Work out the finished part from the listing and answer in its coordinate system (mm). Round coordinates to 2 decimals unless told otherwise and drop trailing zeros. Write each loop counter-clockwise with the first axis right and the second up, starting at its lowest first coordinate (ties: lowest second). Pieces come first, ordered by that corner, then holes.
1. Straight lines are drawn through the part: probe 1 along Y at (x, z) = (0, -0.1); probe 2 along X at (y, z) = (7.5, -0.3); probe 3 along Y at (x, z) = (0.65, -0.05). For each, find the intervals that lie inside material, in ascending order.
2. Find section D-D (y = 5). Write down the section's boundary in (x, z), and give its area (3 significant figures).
3. A flat-ended cylindrical pin translates along its axis: pin 1 Ø0.5 at (y, z) = (6, 0) entering from +X. Find the tip coordinate at first contact, or state that the pin passes through.
4. Find section B-B (y = 0.5). Write down the section's boundary in (x, z), and give its area (3 significant figures).
5. Find section C-C (z = 0.4). Write down the section's boundary in (x, y), and give its area (3 significant figures).
6. Find section A-A (x = 0). Write down the section's boundary in (y, z).
```python
from build123d import *

# Parameters (mm, degrees)
SZKIC1_W                    = 1
SZKIC1_H                    = 1
DODANIE_WYCI_GNI_CIE2_DEPTH = 9.5
SZKIC2_R                    = 0.250044668
WYTNIJ_WYCI_GNI_CIE1_DEPTH  = 9.5
SZKIC3_W                    = 1
SZKIC3_H                    = 1.5
DODANIE_WYCI_GNI_CIE3_DEPTH = 0.5
SZKIC4_W                    = 1
SZKIC4_H                    = 1.498354428
DODANIE_WYCI_GNI_CIE4_DEPTH = 0.5
ZAOKR_GLENIE1_R             = 0.25
ZAOKR_GLENIE2_R             = 0.25


with BuildPart() as part:
    # Szkic1 → Dodanie-wyciągnięcie2 (new body)
    with BuildSketch(Plane(origin=(0, 0, 0), x_dir=(1, 0, 0), z_dir=(0, 1, 0))):
        Rectangle(SZKIC1_W, SZKIC1_H)
    extrude(amount=DODANIE_WYCI_GNI_CIE2_DEPTH)

    # Szkic2 → Wytnij-wyciągnięcie1 (cut)
    with BuildSketch(Plane(origin=(0, 0, -0.5), x_dir=(-1, 0, 0), z_dir=(0, 0, -1))):
        with Locations((0, 0.5)):
            Circle(SZKIC2_R)
    extrude(amount=-WYTNIJ_WYCI_GNI_CIE1_DEPTH, mode=Mode.SUBTRACT)

    # Szkic3 → Dodanie-wyciągnięcie3 (add)
    with BuildSketch(Plane(origin=(0.5, 0, 0), x_dir=(0, 0, -1), z_dir=(1, 0, 0))):
        with Locations((0, 8.75)):
            Rectangle(SZKIC3_W, SZKIC3_H)
    extrude(amount=DODANIE_WYCI_GNI_CIE3_DEPTH)

    # Szkic4 → Dodanie-wyciągnięcie4 (add)
    with BuildSketch(Plane.ZY.offset(0.5)):
        with Locations((0, 8.750822786)):
            Rectangle(SZKIC4_W, SZKIC4_H)
    extrude(amount=DODANIE_WYCI_GNI_CIE4_DEPTH)

    # Zaokrąglenie1
    zaokr_glenie1_edges = [part.edges().sort_by_distance(p)[0] for p in [
        (0, 9.5, -0.5),
        (0.75, 8, 0.5),
        (0.75, 8, -0.5),
        (1, 8.75, 0.5),
        (1, 8.75, -0.5),
        (1, 9.5, 0),
        (-0.75, 8.001645572, -0.5),
        (-1, 8.750822786, -0.5),
        (-1, 8.750822786, 0.5),
        (-1, 9.5, 0),
        (0, 9.5, 0.5),
    ]]
    fillet(zaokr_glenie1_edges, radius=ZAOKR_GLENIE1_R)

    # Zaokrąglenie2
    # the kernel refuses this fillet: 0.25 mm, written as the material it takes off along each edge
    with BuildSketch(Plane(origin=(0.75, 8.25, -0.25), x_dir=(0, -1, 0), z_dir=(1, 0, 0))) as zaokr_glenie2_piece_1_section:
        Polygon((0, 0), (ZAOKR_GLENIE2_R, 0), (ZAOKR_GLENIE2_R, ZAOKR_GLENIE2_R), (0, ZAOKR_GLENIE2_R), align=None)
    zaokr_glenie2_piece_1 = extrude(amount=ZAOKR_GLENIE2_R, mode=Mode.PRIVATE)
    zaokr_glenie2_piece_1 = zaokr_glenie2_piece_1 - Plane(origin=(0.75, 8.25, -0.25), x_dir=(0, 0.7071067811865475, 0.7071067811865475), z_dir=(1, 0, 0)) * Sphere(ZAOKR_GLENIE2_R, mode=Mode.PRIVATE)
    add(zaokr_glenie2_piece_1, mode=Mode.SUBTRACT)
    with BuildSketch(Plane(origin=(-0.75, 8.251645572, -0.25), x_dir=(0, -1, 0), z_dir=(-1, 0, 0))) as zaokr_glenie2_piece_2_section:
        Polygon((0, 0), (ZAOKR_GLENIE2_R, 0), (ZAOKR_GLENIE2_R, -ZAOKR_GLENIE2_R), (0, -ZAOKR_GLENIE2_R), align=None)
    zaokr_glenie2_piece_2 = extrude(amount=ZAOKR_GLENIE2_R, mode=Mode.PRIVATE)
    zaokr_glenie2_piece_2 = zaokr_glenie2_piece_2 - Plane(origin=(-0.75, 8.251645572, -0.25), x_dir=(0, 0.7071067811865475, 0.7071067811865475), z_dir=(-1, 0, 0)) * Sphere(ZAOKR_GLENIE2_R, mode=Mode.PRIVATE)
    add(zaokr_glenie2_piece_2, mode=Mode.SUBTRACT)
    with BuildSketch(Plane(origin=(0.75, 8.25, 0.25), x_dir=(0, -1, 0), z_dir=(1, 0, 0))) as zaokr_glenie2_piece_3_section:
        Polygon((0, 0), (ZAOKR_GLENIE2_R, 0), (ZAOKR_GLENIE2_R, -ZAOKR_GLENIE2_R), (0, -ZAOKR_GLENIE2_R), align=None)
    zaokr_glenie2_piece_3 = extrude(amount=ZAOKR_GLENIE2_R, mode=Mode.PRIVATE)
    zaokr_glenie2_piece_3 = zaokr_glenie2_piece_3 - Plane(origin=(0.75, 8.25, 0.25), x_dir=(0, 0.7071067811865475, -0.7071067811865475), z_dir=(1, 0, 0)) * Sphere(ZAOKR_GLENIE2_R, mode=Mode.PRIVATE)
    add(zaokr_glenie2_piece_3, mode=Mode.SUBTRACT)
    with BuildSketch(Plane(origin=(-1, 8.001645572, 0.25), x_dir=(0, 1, 0), z_dir=(0, 0, -1)), Plane(origin=(1, 8, -0.25), x_dir=(0, 1, 0), z_dir=(0, 0, 1))) as zaokr_glenie2_piece_4:
        with BuildLine():
            CenterArc((ZAOKR_GLENIE2_R, ZAOKR_GLENIE2_R), ZAOKR_GLENIE2_R, 180, 90)
            Line((0, ZAOKR_GLENIE2_R), (0, 0))
            Line((0, 0), (ZAOKR_GLENIE2_R, 0))
        make_face()
    extrude(amount=0.5, mode=Mode.SUBTRACT)
    with BuildSketch(Plane(origin=(-0.5, 8.001645572, 0.5), x_dir=(0, 1, 0), z_dir=(-1, 0, 0))) as zaokr_glenie2_piece_5:
        with BuildLine():
            CenterArc((ZAOKR_GLENIE2_R, ZAOKR_GLENIE2_R), ZAOKR_GLENIE2_R, 180, 90)
            Line((0, ZAOKR_GLENIE2_R), (0, 0))
            Line((0, 0), (ZAOKR_GLENIE2_R, 0))
        make_face()
    extrude(amount=0.25, mode=Mode.SUBTRACT)
    with BuildSketch(Plane(origin=(-0.75, 8.001645572, 0.25), x_dir=(0, 0, 1), z_dir=(1, 0, 0))) as zaokr_glenie2_piece_6:
        with BuildLine():
            CenterArc((0.25 - ZAOKR_GLENIE2_R, -ZAOKR_GLENIE2_R), ZAOKR_GLENIE2_R, 0, 90)
            Line((0.25 - ZAOKR_GLENIE2_R, 0), (0.25, 0))
            Line((0.25, 0), (0.25, -ZAOKR_GLENIE2_R))
        make_face()
    revolve(axis=Axis((-0.75, 8.001645572, 0.25), (0, -1, 0)), revolution_arc=90, mode=Mode.SUBTRACT)


solid = part.part
```
Worked answers:
1. probe 1: y = 0 to 0.25, 0.75 to 9.5
1. probe 2: x = -0.5 to 0.5
1. probe 3: y = 8 to 9.5
2. outline: (-0.5, -0.5) - (0.5, -0.5) - (0.5, 0.5) - (-0.5, 0.5) - close
2. area: 1.00 mm2
3. pin 1: stops at x = 0.5
4. outline: (-0.5, -0.5) - (-0.25, -0.5) - (-0.25, 0.5) - (-0.5, 0.5) - close; (0.25, -0.5) - (0.5, -0.5) - (0.5, 0.5) - (0.25, 0.5) - close
4. area: 0.500 mm2
5. outline: (-0.95, 8.25) arc R0.2 ccw to (-0.75, 8.05) - (-0.5, 8.05) - (-0.5, 0) - (0.5, 0) - (0.5, 8.05) - (0.75, 8.05) arc R0.2 ccw to (0.95, 8.25) - (0.95, 9.25) arc R0.2 ccw to (0.75, 9.45) - (-0.75, 9.45) arc R0.2 ccw to (-0.95, 9.25) - close; hole circle Ø0.5 at (0, 0.5)
5. area: 10.5 mm2
6. outline: (0, -0.5) - (0.25, -0.5) - (0.25, 0.5) - (0, 0.5) - close; (0.75, -0.5) - (9.25, -0.5) arc R0.25 ccw to (9.5, -0.25) - (9.5, 0.25) arc R0.25 ccw to (9.25, 0.5) - (0.75, 0.5) - close
